from build123d import *

# Parameters (mm, degrees)
CROQUIS1_R              = 8
CROQUIS1_R_2            = 0.76
CROQUIS1_W              = 3.2
CROQUIS1_H              = 2.2
SALIENTE_EXTRUIR1_DEPTH = 2
CORTAR_EXTRUIR1_START   = -10
CORTAR_EXTRUIR1_DEPTH   = 10


with BuildPart() as part:
    # Croquis1 → Saliente-Extruir1 (new body)
    with BuildSketch(Plane(origin=(0, 0, 0), x_dir=(1, 0, 0), z_dir=(0, 1, 0))):
        with BuildLine():
            Line((0, 0), (8, 0))
            ThreePointArc((8, 0), (16.485281374, 3.514718626), (20, 12))
            Line((20, 12), (20, 13))
            ThreePointArc((20, 13), (16.778174593, 20.778174593), (9, 24))
            Line((9, 24), (0, 24))
            Line((0, 24), (0, 0))
        make_face()
        with Locations(Location((10, 14, 0), (0, 0, 270))):
            Circle(CROQUIS1_R, mode=Mode.SUBTRACT)
        with Locations(Location((1.67, 22.6, 0), (0, 0, 270))):
            Circle(CROQUIS1_R_2, mode=Mode.SUBTRACT)
        with Locations(Location((1.67, 5.4, 0), (0, 0, 90))):
            Circle(CROQUIS1_R_2, mode=Mode.SUBTRACT)
        with Locations((10, 2.35)):
            Rectangle(CROQUIS1_W, CROQUIS1_H, mode=Mode.SUBTRACT)
        with Locations((3, 2.35)):
            Rectangle(CROQUIS1_W, CROQUIS1_H, mode=Mode.SUBTRACT)
    extrude(amount=SALIENTE_EXTRUIR1_DEPTH)

    # Croquis2 → Cortar-Extruir1 (cut)
    with BuildSketch(Plane(origin=(0, 2, 0), x_dir=(1, 0, 0), z_dir=(0, 1, 0)).offset(CORTAR_EXTRUIR1_START)):
        with BuildLine():
            Line((14.418335952, 26.139278259), (12.736161147, 21.517540966))
            ThreePointArc((12.736161147, 21.517540966), (18, 14), (12.736161147, 6.482459034))
            Line((12.736161147, 6.482459034), (14.418335952, 1.860721741))
            ThreePointArc((14.418335952, 1.860721741), (22.918350097, 14), (14.418335952, 26.139278259))
        make_face()
    extrude(amount=CORTAR_EXTRUIR1_DEPTH, mode=Mode.SUBTRACT)


solid = part.part
Check sheet for the modelled part. Datum: model origin and axes. Units: mm. A direction names the side the tool comes from. Round coordinates to 2 decimals unless told otherwise and drop trailing zeros. Loops run counter-clockwise (first coordinate to the right, second up) from the corner with the lowest first, then second, coordinate; pieces in that order, holes last. Notation, with made-up numbers: M 12,-21 L 49,-21 A24 ccw 49,9 Z; hole C 36,-13 d8. An arc over 180 degrees is marked long. One line per question, with ' | ' between items. Start each with the question number.
Item 1: Section check D-D (x = 10). Record the boundary of the cut face in (y, z), and give its area (3 significant figures).
Item 2: Scan lines: probe 1 along Z at (x, y) = (4, 0.5); probe 2 along Z at (x, y) = (4.5, 1.6); probe 3 along X at (y, z) = (1.1, -5.4). Record each from-to range of solid material in increasing order.
Item 3: Set-up check for faces 1 (the face through (4.6, 1, -2)), 2 (the face through (2, 2, -10)), 3 (the face through (13.565, 0.986, -4.204)): record each of +Z, -Z, +X, -X, +Y, -Y from which the full face is reachable in a straight line by a thin tool's end or side.
Item 4: Release check for a two-part mould opening along Z. For faces 4 (the face through (2, 0, -10)), 5 (the face through (11.23, 0.99, -23.77)), 6 (the face through (3, 1, -1.25)), 7 (the face through (10, 1, -1.25)) record: released by +Z, released by -Z, zero draft, split by the parting line, or undercut.
Item 5: Section check B-B (y = 0.95). Record the boundary of the cut face in (x, z).
Item 6: Section check A-A (x = 1.67). Record the boundary of the cut face in (y, z), and give its area (3 significant figures).
Item 7: Gauge pin test, flat end, axial feed: pin 1 Ø8 at (x, z) = (10.5, -14.5) entering from -Y. Record the tip position at first contact, or that the pin passes through.
Item 8: Section check C-C (z = -5.4). Record the boundary of the cut face in (x, y), and give its area (3 significant figures).
Worked out:
1) outline: M 0,-23.95 L 2,-23.95 L 2,-22 L 0,-22 Z; M 0,-6 L 2,-6 L 2,-3.45 L 0,-3.45 Z; M 0,-1.25 L 2,-1.25 L 2,-0.17 L 0,-0.17 Z | area: 11.2 mm^2
2) probe 1: -24 to -19.29, -8.71 to -3.45, -1.25 to 0 | probe 2: -24 to -19.81, -8.19 to -3.45, -1.25 to 0 | probe 3: 0 to 0.91, 2.43 to 13.13
3) face 1: +Y, -Y | face 2: +Z, -Z, +X, -X, +Y | face 3: +X, +Y, -Y
4) face 4: zero draft | face 5: released by -Z | face 6: undercut | face 7: undercut
5) outline: M 0,-24 L 9,-24 A11 ccw 13.32,-23.12 L 12.74,-21.52 A8 cw long 12.74,-6.48 L 14.42,-1.86 A12 ccw 8,0 L 0,0 Z; hole C 1.67,-22.6 d1.52; hole C 1.67,-5.4 d1.52; hole M 1.4,-3.45 L 4.6,-3.45 L 4.6,-1.25 L 1.4,-1.25 Z; hole M 8.4,-3.45 L 11.6,-3.45 L 11.6,-1.25 L 8.4,-1.25 Z
6) outline: M 0,-24 L 2,-24 L 2,-23.36 L 0,-23.36 Z; M 0,-21.84 L 2,-21.84 L 2,-6.16 L 0,-6.16 Z; M 0,-4.64 L 2,-4.64 L 2,-3.45 L 0,-3.45 Z; M 0,-1.25 L 2,-1.25 L 2,0 L 0,0 Z | area: 37.5 mm^2
7) pin 1: through
8) outline: M 0,0 L 0.91,0 L 0.91,2 L 0,2 Z; M 2.43,0 L 13.13,0 L 13.13,2 L 2.43,2 Z | area: 23.2 mm^2
